Geometry check sheet. Reference: the model listing, model coordinates, mm. Coordinates: 2 decimals unless noted, no trailing zeros. Order: outer loops, then holes, each group sorted by start corner. A loop starts at its lowest first (then second) coordinate and runs counter-clockwise, first axis right, second up. Notation, with made-up numbers: (68, -11) - (73, -11) arc R16 ccw to (73, 3) - close; hole circle Ø7 at (0.25, 61). An arc over 180 degrees is marked (long way). Put each result on its own line as item: value.
from build123d import *


with BuildPart() as f1:
    # F0 (on Front) → F1 (revolve)
    with BuildSketch(Plane.XZ):
        Polygon((0, 3.0734), (0, 0), (25.4, 0), (41.024185, 31.24837), (44.498579, 38.197157), (47.382554, 43.965108), (50.8, 50.8), (47.363834, 50.8), (23.500534, 3.0734), align=None)
        with BuildLine():
            Line((47.382554, 43.965108), (44.498579, 38.197157))
            ThreePointArc((44.498579, 38.197157), (46.627971, 40.737431), (47.382554, 43.965108))
        make_face()
        with BuildLine():
            Line((44.498579, 38.197157), (41.024185, 31.24837))
            ThreePointArc((41.024185, 31.24837), (43.789655, 34.208627), (44.498579, 38.197157))
        make_face()
    revolve(axis=Axis((0, 0, 25.4), (0, 0, 1)))


solid = f1.part
Q1. Draft check along X on faces 1 (the flat face through (0, 0, 3.073)), 2 (the flat face through (-42, 23, 50.8)), 3 (the conical face through (-5.92, -26.66, 10.69)), 4 (the conical face through (45.4, 14.3, 44.4)). Enter one of: pulls with the +X half, pulls with the -X half, needs draft (parallel to the pull), parting line crosses it, or undercut.
Answer block:
face 1: undercut
face 2: needs draft
face 3: undercut
face 4: parting line crosses it
Q2. Section check B-B on y = 0. Record the boundary of the cut face in (x, z).
Answer block:
outline: (-50.8, 50.8) - (-47.38, 43.97) arc R7.15 ccw to (-44.5, 38.2) arc R7.14 ccw to (-41.02, 31.25) - (-25.4, 0) - (25.4, 0) - (41.02, 31.25) arc R7.14 ccw to (44.5, 38.2) arc R7.15 ccw to (47.38, 43.97) - (50.8, 50.8) - (47.36, 50.8) - (23.5, 3.07) - (-23.5, 3.07) - (-47.36, 50.8) - close
Q3. Thickness scan on L1, parallel to Y at x = 17, z = 42; L2, parallel to Y at x = -7, z = 25; L3, parallel to Z at x = 7.5, y = -16. Record the ranges inside material, lowest first. Write a range as [from, to].
Answer block:
L1: y = [-43.94, -39.46], [39.46, 43.94]
L2: y = [-37.25, -33.75], [33.75, 37.25]
L3: z = [0, 3.07]
Q4. Section check D-D on z = 11. Record the boundary of the cut face in (x, y).
Answer block:
outline: circle Ø61.8 at (0, 0); hole circle Ø54.93 at (0, 0)
Q5. Section check A-A on z = 24.5. Record the boundary of the cut face in (x, y).
Answer block:
outline: circle Ø75.3 at (0, 0); hole circle Ø68.43 at (0, 0)
Q6. Depth check by flat-ended pin: pin 1 Ø8 at (x, y) = (3, 22.5) entering from +Z; pin 2 Ø5 at (x, y) = (21, 28.5) entering from +Z; pin 3 Ø1.5 at (y, z) = (-8.5, 44) entering from +X; pin 4 Ø8 at (x, z) = (39.5, 10.5) entering from +Y. Enter the tip coordinate at first touch or a pass-through.
Answer block:
pin 1: stops at z = 9.47
pin 2: stops at z = 31.87
pin 3: stops at x = 47.04
pin 4: passes through
